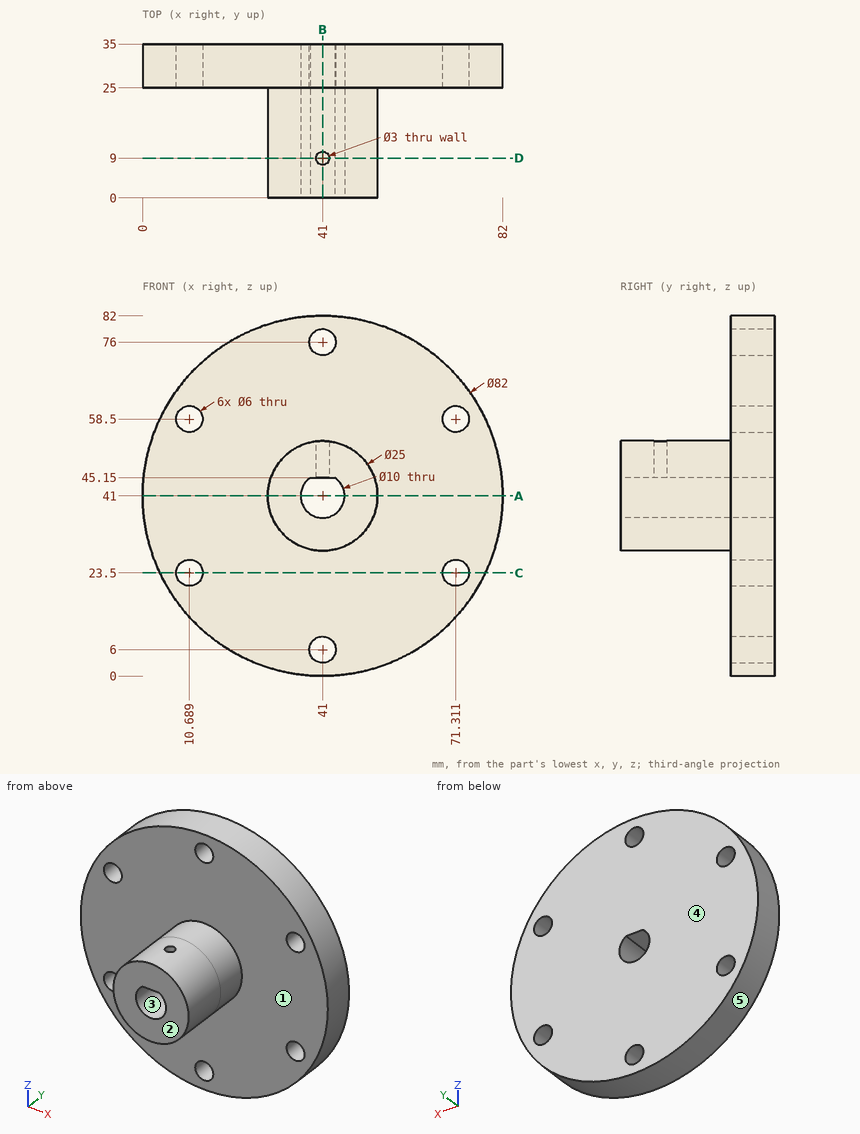
Print and shaded views of the part. All mm, measured from the part's lowest x, y and z. A direction names the side the tool comes from. Coordinates: 2 decimals unless noted, no trailing zeros. Order: outer loops, then holes, each group sorted by start corner. A loop starts at its lowest first (then second) coordinate and runs counter-clockwise, first axis right, second up. Notation, with made-up numbers: (59, -9.5) - (106, -9.5) arc R32 cw to (106, 16.5) - close; hole circle Ø6 at (-6, -33). An arc over 180 degrees is marked (long way). Put each result on its own line as item: value.
1. Tool access for the marked faces 1 and 2: list every direction of +Z, -Z, +X, -X, +Y, -Y with a clear straight run to the whole face (end or side of a thin tool).
Answer sheet:
face 1: -Y
face 2: +Z, -Z, +X, -X, -Y
2. Drop flat-ended pins along their axis: P1, Ø6, axis at y = 22.5, z = 62.5, coming from the +X side; P2, Ø9.5, axis at x = 71.31, z = 23.5, coming from the -Y side; P3, Ø6, axis at x = 39.5, y = 11.5, coming from the -Z side. Give the stop position or say it passes through.
Answer sheet:
P1: stops at x = 76.88
P2: stops at y = 25
P3: stops at z = 28.5
3. Saw through at B-B (x = 41). Write the cut outline in (y, z), and give its area (3 significant figures).
Answer sheet:
outline: (0, 28.5) - (25, 28.5) - (25, 9) - (35, 9) - (35, 36) - (0, 36) - close; (0, 45.15) - (7.5, 45.15) - (7.5, 53.5) - (0, 53.5) - close; (10.5, 45.15) - (35, 45.15) - (35, 73) - (25, 73) - (25, 53.5) - (10.5, 53.5) - close; (25, 0) - (35, 0) - (35, 3) - (25, 3) - close; (25, 79) - (35, 79) - (35, 82) - (25, 82) - close
area: 980 mm^2
4. Saw through at C-C (z = 23.5). Write the cut outline in (x, y), and give its area (3 significant figures).
Answer sheet:
outline: (3.92, 25) - (7.69, 25) - (7.69, 35) - (3.92, 35) - close; (13.69, 25) - (68.31, 25) - (68.31, 35) - (13.69, 35) - close; (74.31, 25) - (78.08, 25) - (78.08, 35) - (74.31, 35) - close
area: 622 mm^2
5. Saw through at A-A (z = 41). Write the cut outline in (x, y), and give its area (4 significant figures).
Answer sheet:
outline: (0, 25) - (28.5, 25) - (28.5, 0) - (36, 0) - (36, 35) - (0, 35) - close; (46, 0) - (53.5, 0) - (53.5, 25) - (82, 25) - (82, 35) - (46, 35) - close
area: 1,095 mm^2
6. Probe line 1 along Y through (x, z) = (41, 50); line 2 along X through (y, z) = (29, 60); line 3 along Z through (x, y) = (71, 33). List the from-to ranges inside material, lowest first. Write a range as [from, to].
Answer sheet:
line 1: y = [0, 7.5], [10.5, 35]
line 2: x = [4.67, 8.09], [13.29, 68.71], [73.91, 77.33]
line 3: z = [13.05, 20.52], [26.48, 55.52], [61.48, 68.95]
7. Saw through at D-D (y = 9). Write the cut outline in (x, z), and give its area (3 significant figures).
Answer sheet:
outline: (38.21, 45.15) - (39.5, 45.15) - (39.5, 53.41) arc R12.5 ccw (long way) to (42.5, 53.41) - (42.5, 45.15) - (43.79, 45.15) arc R5 cw (long way) to start
area: 391 mm^2
8. Pull direction X, two halves, no side cores. Call the marked faces 3, 4 and 5: pulls with the +X half, pulls with the -X half, needs draft (parallel to the pull), parting line crosses it, or undercut.
Answer sheet:
face 3: undercut
face 4: needs draft
face 5: parting line crosses it
